```python
from build123d import *

# Parameters (mm, degrees)
SKETCH1_W           = 50
SKETCH1_H           = 30
SKETCH1_R           = 3
BOSS_EXTRUDE1_DEPTH = 1.5
FILLET1_R           = 2.5
SKETCH2_R           = 7.8
BOSS_EXTRUDE2_DEPTH = 4


with BuildPart() as part:
    # Sketch1 → Boss-Extrude1 (new body, symmetric)
    with BuildSketch(Plane.XY):
        Rectangle(SKETCH1_W, SKETCH1_H)
        with Locations((-17.5, 0)):
            Circle(SKETCH1_R, mode=Mode.SUBTRACT)
        with Locations((17.5, 0)):
            Circle(SKETCH1_R, mode=Mode.SUBTRACT)
    extrude(amount=BOSS_EXTRUDE1_DEPTH, both=True)

    # Fillet1
    fillet1_edges = [part.edges().sort_by_distance(p)[0] for p in [
        (-25, 15, 0),
        (25, 15, 0),
        (25, -15, 0),
        (-25, -15, 0),
    ]]
    fillet(fillet1_edges, radius=FILLET1_R)

    # Sketch2 → Boss-Extrude2 (add)
    with BuildSketch(Plane.XY.offset(1.5)):
        with BuildLine():
            Line((7.5, -10), (-7.5, -10))
            ThreePointArc((-7.5, -10), (-9.267766953, -9.267766953), (-10, -7.5))
            Line((-10, -7.5), (-10, 7.5))
            ThreePointArc((-10, 7.5), (-9.267766953, 9.267766953), (-7.5, 10))
            Line((-7.5, 10), (7.5, 10))
            ThreePointArc((7.5, 10), (9.267766953, 9.267766953), (10, 7.5))
            Line((10, 7.5), (10, -7.5))
            ThreePointArc((10, -7.5), (9.267766953, -9.267766953), (7.5, -10))
        make_face()
        Circle(SKETCH2_R, mode=Mode.SUBTRACT)
    extrude(amount=BOSS_EXTRUDE2_DEPTH)


solid = part.part
```
The model under review builds one solid part; all positions refer to its coordinate system, in mm. A direction names the side the tool comes from. Give positions to 0.01 mm unless a question says otherwise; leave off trailing zeros. Write each loop counter-clockwise with the first axis right and the second up, starting at its lowest first coordinate (ties: lowest second). Pieces come first, ordered by that corner, then holes. Notation, with made-up numbers: (51.5, -6) - (69.5, -6) arc R17 ccw to (69.5, 2) - close; hole circle Ø10 at (-9.5, -14). An arc over 180 degrees is marked (long way). Answer in a Markdown table with one row per item. Add a question column.
1. Tool access review of faces 1 (the flat face through (0, 0, 1.5)), 2 (the flat face through (10, 0, 3)), 3 (the flat face through (0, 10, 3)), 4 (the cylindrical face through (9.248, 9.287, 3.472)), 5 (the cylindrical face through (-9.248, -9.287, 3.472)): name each direction out of +Z, -Z, +X, -X, +Y, -Y from which nothing blocks a thin tool from reaching the whole face with its end or side.
2. We need section B-B on y = 0. Write out the cut boundary in (x, z).
3. We need section D-D on y = -6.5. Write out the cut boundary in (x, z).
4. Insertion check: P1, Ø3, axis at x = 3, z = 3.5, coming from the +Y side. The pin has a flat end and moves straight along its axis. Give the tip position at first contact, or say it passes through.
5. Wall thickness on line 1 along Y through (x, z) = (-17.5, -0.8); line 2 along Y through (x, z) = (0, 2.65); line 3 along X through (y, z) = (-2.75, 0): over which ranges is each line inside the solid? List them lowest first. Write a range as [from, to].
6. We need section C-C on z = 2. Write out the cut boundary in (x, y).
7. We need section A-A on x = -17.5. Write out the cut boundary in (y, z), then the cut area to 3 significant figures.
8. Draft analysis for pull direction X (two halves, no side actions). For faces 6 (the flat face through (0, -15, 0)), 7 (the cylindrical face through (24.287, 14.248, -0.021)), 8 (the cylindrical face through (15.1, -1.8, 0)), state which applies: +X half, -X half, draft (parallel to the pull), parting line (faces both ways), or undercut.
Ans:
| question | item | result |
|---|---|---|
| 1 | face 1 | +Z |
| 1 | face 2 | +Z, +X, +Y, -Y |
| 1 | face 3 | +Z, +X, -X, +Y |
| 1 | face 4 | +Z, +X, +Y |
| 1 | face 5 | +Z, -X, -Y |
| 2 | outline | (-25, -1.5) - (-20.5, -1.5) - (-20.5, 1.5) - (-25, 1.5) - close; (-14.5, -1.5) - (14.5, -1.5) - (14.5, 1.5) - (10, 1.5) - (10, 5.5) - (7.8, 5.5) - (7.8, 1.5) - (-7.8, 1.5) - (-7.8, 5.5) - (-10, 5.5) - (-10, 1.5) - (-14.5, 1.5) - close; (20.5, -1.5) - (25, -1.5) - (25, 1.5) - (20.5, 1.5) - close |
| 3 | outline | (-25, -1.5) - (25, -1.5) - (25, 1.5) - (10, 1.5) - (10, 5.5) - (4.31, 5.5) - (4.31, 1.5) - (-4.31, 1.5) - (-4.31, 5.5) - (-10, 5.5) - (-10, 1.5) - (-25, 1.5) - close |
| 4 | P1 | stops at y = 10 |
| 5 | line 1 | y = [-15, -3], [3, 15] |
| 5 | line 2 | y = [-10, -7.8], [7.8, 10] |
| 5 | line 3 | x = [-25, -18.7], [-16.3, 16.3], [18.7, 25] |
| 6 | outline | (-10, -7.5) arc R2.5 ccw to (-7.5, -10) - (7.5, -10) arc R2.5 ccw to (10, -7.5) - (10, 7.5) arc R2.5 ccw to (7.5, 10) - (-7.5, 10) arc R2.5 ccw to (-10, 7.5) - close; hole circle Ø15.6 at (0, 0) |
| 7 | outline | (-15, -1.5) - (-3, -1.5) - (-3, 1.5) - (-15, 1.5) - close; (3, -1.5) - (15, -1.5) - (15, 1.5) - (3, 1.5) - close |
| 7 | area | 72.0 mm^2 |
| 8 | face 6 | draft |
| 8 | face 7 | +X half |
| 8 | face 8 | undercut |
